Part model, mm, in its own coordinate system. A direction names the side the tool comes from. Round coordinates to 2 decimals unless told otherwise and drop trailing zeros. Order: outer loops, then holes, each group sorted by start corner. A loop starts at its lowest first (then second) coordinate and runs counter-clockwise, first axis right, second up. Notation, with made-up numbers: (-22, 5.25) - (3, 5.25) arc R23 ccw to (3, 29.25) - close; hole circle Ø4 at (41, 51.25). An arc over 180 degrees is marked (long way). Answer as a JSON object with one key per item and string values.
Autodesk Inventor part; units mm, degrees
ref_plane "YZ Plane" through (0, 0, 0) normal (1, 0, 0) x (0, 1, 0)
ref_plane "XZ Plane" through (0, 0, 0) normal (0, 1, 0) x (-1, 0, 0)
ref_plane "XY Plane" through (0, 0, 0) normal (0, 0, 1) x (1, 0, 0)
sketch "Sketch1" plane through (0, 0, 0) normal (0, 0, 1) x (1, 0, 0)
  circle A0 centre (0, 0) radius 52
  circle A1 centre (0, 0) radius 62.5
  dimension "d0" = 125
  dimension "d1" = 104
extrude "Extrusion1" add sketch "Sketch1" along normal blind 400
sketch "Sketch2" plane through (0, 0, 0) normal (0, 1, 0) x (-1, 0, 0)
  line L0 (62.5, 400) -> (-62.5, 400)
  line L1 (62.5, 0) -> (-62.5, 0)
  line L2 (-62.5, 280) -> (-12.5, 280)
  line L3 (-12.5, 280) -> (-12.5, 210)
  line L4 (-12.5, 210) -> (-62.5, 181.1325)
  line L5 (-62.5, 0) -> (-62.5, 400)
  point P0 (0, 0)
  dimension "d4" = 60
  dimension "d5" = 50
  dimension "d6" = 120
  dimension "d7" = 70
extrude "Extrusion2" cut sketch "Sketch2" along normal through all both and the other way through all
properties part number "NVPH-341 second tube"
Item 1: Cut at D-D (z = 315). Write the cut outline in (x, y).
Taken from the geometry:
{"outline": "circle Ø125 at (0, 0); hole circle Ø104 at (0, 0)"}
Item 2: Tool access for faces 5 (the flat face through (52, -5, 280)), 6 (the cylindrical face through (-51.95, -2.29, 197.2)): list every direction of +Z, -Z, +X, -X, +Y, -Y with a clear straight run to the whole face (end or side of a thin tool).
Taken from the geometry:
{"face 5": "+X, +Y, -Y", "face 6": "+Z, -Z"}
Item 3: Cut at C-C (x = 24). Write the cut outline in (y, z), plus the area to 3 significant figures.
Taken from the geometry:
{"outline": "(-57.71, 0) - (-46.13, 0) - (-46.13, 203.36) - (-57.71, 203.36) - close; (-57.71, 280) - (-46.13, 280) - (-46.13, 400) - (-57.71, 400) - close; (46.13, 0) - (57.71, 0) - (57.71, 203.36) - (46.13, 203.36) - close; (46.13, 280) - (57.71, 280) - (57.71, 400) - (46.13, 400) - close", "area": "7,490 mm2"}
Item 4: Probe L1, parallel to Y at x = 1.5, z = 187.5; L2, parallel to X at y = 3, z = 60.5; L3, parallel to Y at x = -38.5, z = 370. List the from-to ranges inside material, lowest first. Write a range as from..to.
Taken from the geometry:
{"L1": "-62.48..-51.98, 51.98..62.48", "L2": "-62.43..-51.91, 51.91..62.43", "L3": "-49.23..-34.95, 34.95..49.23"}
Item 5: Two-plate mould, pull along Z, no slides. Class faces 1 (the flat face through (-23, 47, 400)), 2 (the cylindrical face through (-62.44, -2.75, 197.2)), 3 (the flat face through (-23, 47, 0)), 4 (the flat face through (12.5, -56, 245)): pulls with the +Z half, pulls with the -Z half, needs draft (parallel to the pull), parting line crosses it, or undercut.
Taken from the geometry:
{"face 1": "pulls with the +Z half", "face 2": "needs draft", "face 3": "pulls with the -Z half", "face 4": "undercut"}
Item 6: Cut at B-B (y = 25). Write the cut outline in (x, z) (3 decimals).
Taken from the geometry:
{"outline": "(-57.282, 0) - (-45.596, 0) - (-45.596, 400) - (-57.282, 400) - close; (45.596, 0) - (57.282, 0) - (57.282, 184.145) - (45.596, 190.892) - close; (45.596, 280) - (57.282, 280) - (57.282, 400) - (45.596, 400) - close"}
Item 7: Cut at A-A (x = 0). Write the cut outline in (y, z), plus the area to 3 significant figures.
Taken from the geometry:
{"outline": "(-62.5, 0) - (-52, 0) - (-52, 400) - (-62.5, 400) - close; (52, 0) - (62.5, 0) - (62.5, 400) - (52, 400) - close", "area": "8,400 mm2"}
Item 8: Drop flat-ended pins along their axis: P1, Ø4, axis at x = -33.5, z = 200.5, coming from the +Y side; P2, Ø10, axis at x = 44, y = 1, coming from the +Z side; P3, Ø4, axis at y = -38.5, z = 268, coming from the -X side; P4, Ø10, axis at x = 41.5, z = 286.5, coming from the -Y side. Give the stop position or say it passes through.
Taken from the geometry:
{"P1": "y = 53.98", "P2": "through", "P3": "x = -50.73", "P4": "y = -50.73"}
